from build123d import *

# Parameters (mm, degrees)
F1_DEPTH = 35
F2_R     = 10
F3_R     = 5
F4_R     = 12.5
F5_DEPTH = 85.001


with BuildPart() as f1:
    # F0 (on Front) → F1 (new body, symmetric)
    with BuildSketch(Plane.XZ):
        Polygon((-355, 0), (355, 0), (355, 25), (274.21539, 25), (215, 25), (-175, 25), (-254.970563, 25), (-355, 25), align=None)
        Polygon((215, 25), (274.21539, 25), (303.082904, 75), (355, 75), (355, 85), (295, 85), (267.287187, 37), (215, 37), align=None)
        Polygon((-281.970563, 52), (-254.970563, 25), (-175, 25), (-175, 37), (-250, 37), (-275, 62), (-355, 62), (-355, 52), align=None)
    extrude(amount=F1_DEPTH, both=True)

    # F2
    f2_edges = [f1.edges().sort_by_distance(p)[0] for p in [
        (-175, 0, 37),
        (-250, 0, 37),
        (-281.970563, 0, 52),
        (-275, 0, 62),
        (267.287187, 0, 37),
        (295, 0, 85),
        (303.082904, 0, 75),
        (215, 0, 37),
    ]]
    fillet(f2_edges, radius=F2_R)

    # F3
    f3_edges = [f1.edges().sort_by_distance(p)[0] for p in [
        (-254.970563, 0, 25),
        (274.21539, 0, 25),
    ]]
    fillet(f3_edges, radius=F3_R)

    # F4 (on Top) → F5 (cut, through all)
    with BuildSketch(Plane.XY):
        with Locations((-325, 0)):
            Circle(F4_R)
        with Locations((325, 0)):
            Circle(F4_R)
    extrude(amount=F5_DEPTH, mode=Mode.SUBTRACT)


solid = f1.part
Input: part model. Units: mm. Frame: model coordinates. A direction names the side the tool comes from. Round coordinates to 2 decimals unless told otherwise and drop trailing zeros. Loops run counter-clockwise (first coordinate to the right, second up) from the corner with the lowest first, then second, coordinate; pieces in that order, holes last. Notation, with made-up numbers: M 22,44 L 45,44 A12 ccw 45,64 Z; hole C -14,55.25 d6. An arc over 180 degrees is marked long. Answer as CSV lines item,"result". Start each with the question number.
(1) Section D-D, the plane x = 76.5. Output: boundary loops of the cut face in (y, z).
(2) Line query: line 1 (X direction, y = 0, z = 17.5); line 2 (Y direction, x = -325, z = 57.75); line 3 (Z direction, x = -301, y = -24). Output: solid intervals per line, ascending. Write a range as [from, to].
(3) Section B-B, the plane z = 13.5. Output: boundary loops of the cut face in (x, y).
(4) First-contact query: pin 1 (15 mm diameter, centred on x = -325, y = 0, fed in from +Z); pin 2 (4 mm diameter, centred on y = -22.5, z = 45.5, fed in from +X); pin 3 (18.5 mm diameter, centred on x = 243.5, y = 1, fed in from +Z); pin 4 (21 mm diameter, centred on x = 49.5, y = -10.5, fed in from +Z). Flat tips, straight axial feed; report the tip coordinate or a pass-through.
(5) Reachability of faces 1 (the flat face through (-308, 0, 62)), 2 (the flat face through (289.22, -0.49, 50.99)), 3 (the flat face through (-313, -8, 52)), 4 (the flat face through (23, 0, 25)) from +Z, -Z, +X, -X, +Y, -Y: full face, straight path, thin tool, end or side. Return the list, or none.
(6) Draft query along Z for faces 5 (the flat face through (-310, 0, 25)), 6 (the flat face through (355, 0, 12)), 7 (the flat face through (281.3, -0.49, 61.27)). Return one class per face: released by +Z, released by -Z, zero draft, split by the parting line, or undercut.
(7) Section A-A, the plane x = 325. Output: boundary loops of the cut face in (y, z).
Values found:
1,outline,"M -35,0 L 35,0 L 35,25 L -35,25 Z"
2,line 1,"x = [-355, -337.5], [-312.5, 312.5], [337.5, 355]"
2,line 2,"y = [-35, -12.5], [12.5, 35]"
2,line 3,"z = [0, 25], [52, 62]"
3,outline,"M -355,-35 L 355,-35 L 355,35 L -355,35 Z; hole C -325,0 d25; hole C 325,0 d25"
4,pin 1,"passes through"
4,pin 2,"stops at x = 287.21"
4,pin 3,"stops at z = 37"
4,pin 4,"stops at z = 25"
5,face 1,"+Z, -X, +Y, -Y"
5,face 2,"+X, +Y, -Y"
5,face 3,"-X, +Y, -Y"
5,face 4,"+Z, +Y, -Y"
6,face 5,"undercut"
6,face 6,"zero draft"
6,face 7,"released by +Z"
7,outline,"M -35,0 L -12.5,0 L -12.5,25 L -35,25 Z; M -35,75 L -12.5,75 L -12.5,85 L -35,85 Z; M 12.5,0 L 35,0 L 35,25 L 12.5,25 Z; M 12.5,75 L 35,75 L 35,85 L 12.5,85 Z"
